Can you work these out from the model? Positions are in its coordinate system, mm. A direction names the side the tool comes from. Give positions to 0.01 mm unless a question says otherwise; leave off trailing zeros. Order: outer loops, then holes, each group sorted by start corner. A loop starts at its lowest first (then second) coordinate and runs counter-clockwise, first axis right, second up. Notation, with made-up numbers: M 81,-22 L 138,-22 A17 cw 138,-10 Z; hole C 31,31 d8. An arc over 180 degrees is marked long. Use one line per item in the form item = value. Start each with the question number.
1. We'd pull the mould along X, two halves only. Please class faces 1 (the face through (88, 18.1, -24.5)), 2 (the face through (54.1, 9.5, -1)), 3 (the face through (75.5, -0.6, -1.8)): +X half, -X half, draft (parallel to the pull), parting line (faces both ways), or undercut.
2. I want a section at A-A, the plane y = 13.5. List the corners of the cut face in (x, z) for me, and give its area (3 significant figures).
3. I need wall thicknesses on L1, parallel to Z at x = 65, y = 15; L2, parallel to X at y = 18.75, z = -18.5; L3, parallel to Y at x = 14, z = -1.5. Which ranges of each line are inside material? Lowest first, please.
4. I want a section at B-B, the plane y = 1.75. List the corners of the cut face in (x, z) for me.
5. For faces 4 (the face through (90, 18, -24)), 5 (the face through (50.5, 3, -1)), 6 (the face through (89, 9, -25)), 7 (the face through (43, 12, -2)), 8 (the face through (89, 7, -22)), which set-ups out of +Z, -Z, +X, -X, +Y, -Y let a thin tool reach every point of the face, with its end or its side?
6. Will these pins go through, and if not, where does the flat tip stop? P1, Ø0.5, axis at x = 45, z = -0.5, coming from the -Y side; P2, Ø1.6, axis at y = 6, z = -1, coming from the +X side; P3, Ø2, axis at x = 89.5, y = 3.5, coming from the -Z side.
7. I want a section at C-C, the plane x = 75. List the corners of the cut face in (y, z) for me.
8. I want a section at D-D, the plane z = -26.5. List the corners of the cut face in (x, y) for me.
```python
from build123d import *

# Parameters (mm, degrees)
P_IDAT_VYSUNUT_M1_DEPTH  = 25
SKICA2_W                 = 88
SKICA2_H                 = 1
P_IDAT_VYSUNUT_M2_DEPTH  = 0.6
ODEBRAT_VYSUNUT_M1_REACH = 63
SKICA5_W                 = 10
SKICA5_H                 = 8.6
SKICA5_W_2               = 18
SKICA5_H_2               = 10.6
ODEBRAT_VYSUNUT_M2_REACH = 92
SKICA6_W                 = 16
SKICA6_H                 = 15.6
SKICA6_W_2               = 19
SKICA6_H_2               = 18.6
FILLET1_R                = 2
CUT_EXTRUDE2_REACH       = 92
SKETCH2_W                = 1
SKETCH2_H                = 18.6


with BuildPart() as part:
    # Skica1 → Přidat vysunutím1 (new body)
    with BuildSketch(Plane(origin=(0, 0, 0), x_dir=(1, 0, 0), z_dir=(0, 1, 0))):
        Polygon((88, 2), (90, 2), (90, 60), (89, 60), (89, 61), (88, 61), align=None)
        Polygon((1, 1), (1, 0), (90, 0), (90, 2), (88, 2), (0, 2), (0, 1), align=None)
    extrude(amount=P_IDAT_VYSUNUT_M1_DEPTH)

    # Skica2 → Přidat vysunutím2 (add)
    with BuildSketch(Plane.XZ):
        with Locations((44, -1.5)):
            Rectangle(SKICA2_W, SKICA2_H)
        Polygon((89, -1), (88, -1), (88, -2), (88, -61), (89, -61), align=None)
    extrude(amount=P_IDAT_VYSUNUT_M2_DEPTH)

    # Skica5 → Odebrat vysunutím1 (cut, up to next)
    with BuildSketch(Plane.XY, mode=Mode.PRIVATE) as odebrat_vysunut_m1_sk1:
        with Locations((11, 3.7)):
            Rectangle(SKICA5_W, SKICA5_H)
    odebrat_vysunut_m1_tool1 = extrude(odebrat_vysunut_m1_sk1.sketch, amount=-ODEBRAT_VYSUNUT_M1_REACH, mode=Mode.PRIVATE) & part.part
    add(odebrat_vysunut_m1_tool1.solids().sort_by_distance((11, 3.7, 0))[0], mode=Mode.SUBTRACT)
    # Skica5 → Odebrat vysunutím1 (cut, up to next)
    with BuildSketch(Plane.XY, mode=Mode.PRIVATE) as odebrat_vysunut_m1_sk2:
        with Locations((33, 4.7)):
            Rectangle(SKICA5_W_2, SKICA5_H_2)
    odebrat_vysunut_m1_tool2 = extrude(odebrat_vysunut_m1_sk2.sketch, amount=-ODEBRAT_VYSUNUT_M1_REACH, mode=Mode.PRIVATE) & part.part
    add(odebrat_vysunut_m1_tool2.solids().sort_by_distance((33, 4.7, 0))[0], mode=Mode.SUBTRACT)
    # Skica5 → Odebrat vysunutím1 (cut, up to next)
    with BuildSketch(Plane.XY, mode=Mode.PRIVATE) as odebrat_vysunut_m1_sk3:
        with BuildLine():
            Line((50.5, 6), (50.5, -0.6))
            Line((50.5, -0.6), (57.5, -0.6))
            Line((57.5, -0.6), (57.5, 6))
            ThreePointArc((57.5, 6), (54, 9.5), (50.5, 6))
        make_face()
    odebrat_vysunut_m1_tool3 = extrude(odebrat_vysunut_m1_sk3.sketch, amount=-ODEBRAT_VYSUNUT_M1_REACH, mode=Mode.PRIVATE) & part.part
    add(odebrat_vysunut_m1_tool3.solids().sort_by_distance((54, 4.107084, 0))[0], mode=Mode.SUBTRACT)

    # Skica6 → Odebrat vysunutím2 (cut, up to next)
    with BuildSketch(Plane(origin=(90, 0, 0), x_dir=(0, 0, -1), z_dir=(1, 0, 0)), mode=Mode.PRIVATE) as odebrat_vysunut_m2_sk1:
        with Locations((14, 7.2)):
            Rectangle(SKICA6_W, SKICA6_H)
    odebrat_vysunut_m2_tool1 = extrude(odebrat_vysunut_m2_sk1.sketch, amount=-ODEBRAT_VYSUNUT_M2_REACH, mode=Mode.PRIVATE) & part.part
    add(odebrat_vysunut_m2_tool1.solids().sort_by_distance((90, 7.2, -14))[0], mode=Mode.SUBTRACT)
    # Skica6 → Odebrat vysunutím2 (cut, up to next)
    with BuildSketch(Plane(origin=(90, 0, 0), x_dir=(0, 0, -1), z_dir=(1, 0, 0)), mode=Mode.PRIVATE) as odebrat_vysunut_m2_sk2:
        with Locations((51.5, 8.7)):
            Rectangle(SKICA6_W_2, SKICA6_H_2)
    odebrat_vysunut_m2_tool2 = extrude(odebrat_vysunut_m2_sk2.sketch, amount=-ODEBRAT_VYSUNUT_M2_REACH, mode=Mode.PRIVATE) & part.part
    add(odebrat_vysunut_m2_tool2.solids().sort_by_distance((90, 8.7, -51.5))[0], mode=Mode.SUBTRACT)
    # Skica6 → Odebrat vysunutím2 (cut, up to next)
    with BuildSketch(Plane(origin=(90, 0, 0), x_dir=(0, 0, -1), z_dir=(1, 0, 0)), mode=Mode.PRIVATE) as odebrat_vysunut_m2_sk3:
        with Locations((33, 8.7)):
            Rectangle(SKICA6_W, SKICA6_H_2)
    odebrat_vysunut_m2_tool3 = extrude(odebrat_vysunut_m2_sk3.sketch, amount=-ODEBRAT_VYSUNUT_M2_REACH, mode=Mode.PRIVATE) & part.part
    add(odebrat_vysunut_m2_tool3.solids().sort_by_distance((90, 8.7, -33))[0], mode=Mode.SUBTRACT)

    # Fillet1
    fillet1_edges = [part.edges().sort_by_distance(p)[0] for p in [
        (90, 12.5, 0),
    ]]
    fillet(fillet1_edges, radius=FILLET1_R)

    # Sketch2 → Cut-Extrude2 (cut, up to next)
    with BuildSketch(Plane(origin=(90, 0, 0), x_dir=(0, 0, -1), z_dir=(1, 0, 0)), mode=Mode.PRIVATE) as cut_extrude2_sk1:
        with Locations((41.5, 8.7)):
            Rectangle(SKETCH2_W, SKETCH2_H)
    cut_extrude2_tool1 = extrude(cut_extrude2_sk1.sketch, amount=-CUT_EXTRUDE2_REACH, mode=Mode.PRIVATE) & part.part
    add(cut_extrude2_tool1.solids().sort_by_distance((90, 8.7, -41.5))[0], mode=Mode.SUBTRACT)


solid = part.part
```
Check result:
q1.face_1 = -X half
q1.face_2 = undercut
q1.face_3 = draft
q2.outline = M 0,-2 L 88,-2 L 88,-6 L 90,-6 L 90,-2 A2 ccw 88,0 L 1,0 L 1,-1 L 0,-1 Z; M 88,-25 L 90,-25 L 90,-22 L 88,-22 Z
q2.area = 192 mm2
q3.L1 = -2 to 0
q3.L2 = 88 to 90
q3.L3 = 8 to 25
q4.outline = M 0,-2 L 6,-2 L 6,0 L 1,0 L 1,-1 L 0,-1 Z; M 16,-2 L 24,-2 L 24,0 L 16,0 Z; M 42,-2 L 50.5,-2 L 50.5,0 L 42,0 Z; M 57.5,-2 L 88,-2 L 88,-6 L 90,-6 L 90,-2 A2 ccw 88,0 L 57.5,0 Z; M 88,-25 L 90,-25 L 90,-22 L 88,-22 Z
q5.face_4 = +Z, -Z, +X, +Y, -Y
q5.face_5 = +Z, -Z, -Y
q5.face_6 = -Z, +X, -X, -Y
q5.face_7 = -Z, -X, +Y, -Y
q5.face_8 = +X, -X, -Y
q6.P1 = 0
q6.P2 = 89.99
q6.P3 = -25
q7.outline = M -0.6,-2 L 25,-2 L 25,0 L 0,0 L 0,-1 L -0.6,-1 Z
q8.outline = M 88,18 L 90,18 L 90,25 L 88,25 Z
